Can you work these out from the model? Positions are in its coordinate system, mm. Give positions to 0.01 mm unless a question says otherwise; leave off trailing zeros. Order: outer loops, then holes, each group sorted by start corner. A loop starts at its lowest first (then second) coordinate and runs counter-clockwise, first axis right, second up. Notation, with made-up numbers: (-37, 16) - (-18, 16) arc R24 ccw to (-18, 32) - close; hole circle Ø9 at (5, 36.5). An arc over 180 degrees is marked (long way). Answer as a JSON object with one key per item and string values.
```python
from build123d import *

# Parameters (mm, degrees)
RESSALTO_EXTRUS_O1_DEPTH                     = 1.5
ESCAREADO_PARA_PARAFUSO_ALLEN_SEXTAV_2_COUNT = 2
ESCAREADO_PARA_PARAFUSO_ALLEN_SEXTAV_2_PITCH = 194
ESCAREADO_PARA_PARAFUSO_ALLEN_SEXTAV_3_COUNT = 2
ESCAREADO_PARA_PARAFUSO_ALLEN_SEXTAV_3_PITCH = 242.881337709
ESCAREADO_PARA_PARAFUSO_ALLEN_SEXTAV_4_COUNT = 2
ESCAREADO_PARA_PARAFUSO_ALLEN_SEXTAV_4_PITCH = 186.909989587


with BuildPart() as part:
    # Esboço1 → Ressalto-extrusão1 (new body)
    with BuildSketch(Plane.XY):
        Polygon((100.860947645, 140.996609125), (-107.139052355, 140.996609125), (-107.139052355, -8.842442963), (-72.139052355, -38.210930054), (-72.139052355, -137.003390875), (65.860947645, -137.003390875), (65.860947645, -38.210930054), (100.860947645, -8.842442963), align=None)
    extrude(amount=RESSALTO_EXTRUS_O1_DEPTH)

    # Esboço3 → Escareado para parafuso Allen sextavado escareado de M41 (revolve, cut)
    with BuildSketch(Plane(origin=(-100.139052355, 95.996609125, 1.5), x_dir=(0, -1, 0), z_dir=(1, 0, 0))):
        Polygon((0, 0), (0, 1.5), (2.25, 1.5), (2.25, 2.23), (4.48, 0), align=None)
    escareado_para_parafuso_allen_sextavado = revolve(axis=Axis((-100.139052355, 95.996609125, 7.85), (0, 0, -1)), mode=Mode.SUBTRACT)

    # Escareado para parafuso Allen sextav 2: Escareado para parafuso Allen sextavado escareado de M41 ×2
    with Locations(*[(i * ESCAREADO_PARA_PARAFUSO_ALLEN_SEXTAV_2_PITCH, 0, 0) for i in range(1, ESCAREADO_PARA_PARAFUSO_ALLEN_SEXTAV_2_COUNT)]):
        add(escareado_para_parafuso_allen_sextavado, mode=Mode.SUBTRACT)

    # Escareado para parafuso Allen sextav 3: Escareado para parafuso Allen sextavado escareado de M41 ×2
    with Locations(*[Vector(0.654640663, -0.755940211, 0) * (i * ESCAREADO_PARA_PARAFUSO_ALLEN_SEXTAV_3_PITCH) for i in range(1, ESCAREADO_PARA_PARAFUSO_ALLEN_SEXTAV_3_COUNT)]):
        add(escareado_para_parafuso_allen_sextavado, mode=Mode.SUBTRACT)

    # Escareado para parafuso Allen sextav 4: Escareado para parafuso Allen sextavado escareado de M41 ×2
    with Locations(*[Vector(0.187255909, -0.982311165, 0) * (i * ESCAREADO_PARA_PARAFUSO_ALLEN_SEXTAV_4_PITCH) for i in range(1, ESCAREADO_PARA_PARAFUSO_ALLEN_SEXTAV_4_COUNT)]):
        add(escareado_para_parafuso_allen_sextavado, mode=Mode.SUBTRACT)


solid = part.part
```
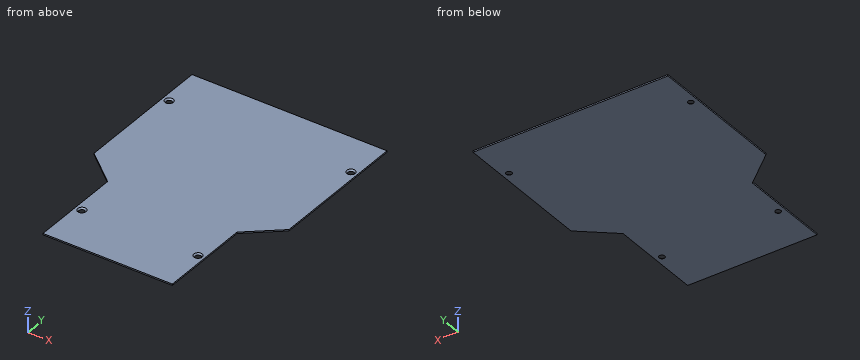
Q1. I'm going to push a flat-ended pin straight in: pin 1 Ø0.8 at (y, z) = (-71.5, 1) entering from +X. Where does the tip first touch, or does it pass through?
Recorded:
{"pin 1": "stops at x = 65.86"}
Q2. If we section it at A-A, the plane z = 0.3: Please give me the cut outline in (x, y), then the cut area to 3 significant figures.
Recorded:
{"outline": "(-107.14, -8.84) - (-72.14, -38.21) - (-72.14, -137) - (65.86, -137) - (65.86, -38.21) - (100.86, -8.84) - (100.86, 141) - (-107.14, 141) - close; hole circle Ø6.56 at (-100.14, 96); hole circle Ø6.56 at (-65.14, -87.61); hole circle Ø6.56 at (58.86, -87.61); hole circle Ø6.56 at (93.86, 96)", "area": "49,700 mm^2"}
Q3. If we section it at C-C, the plane x = -86: Please give me the cut outline in (y, z).
Recorded:
{"outline": "(-26.58, 0) - (141, 0) - (141, 1.5) - (-26.58, 1.5) - close"}
Q4. I need wall thicknesses on L1, parallel to X at y = 94, z = 0.45; L2, parallel to X at y = -98.5, z = 0.7; L3, parallel to Y at x = 75, z = 0.7. Which ranges of each line are inside material? Lowest first, please.
Recorded:
{"L1": "x = -107.14 to -102.93, -97.35 to 91.07, 96.65 to 100.86", "L2": "x = -72.14 to 65.86", "L3": "y = -30.54 to 141"}
Q5. If we section it at B-B, the plane y = -113: Please give me the cut outline in (x, z), then the cut area to 3 significant figures.
Recorded:
{"outline": "(-72.14, 0) - (65.86, 0) - (65.86, 1.5) - (-72.14, 1.5) - close", "area": "207 mm^2"}
